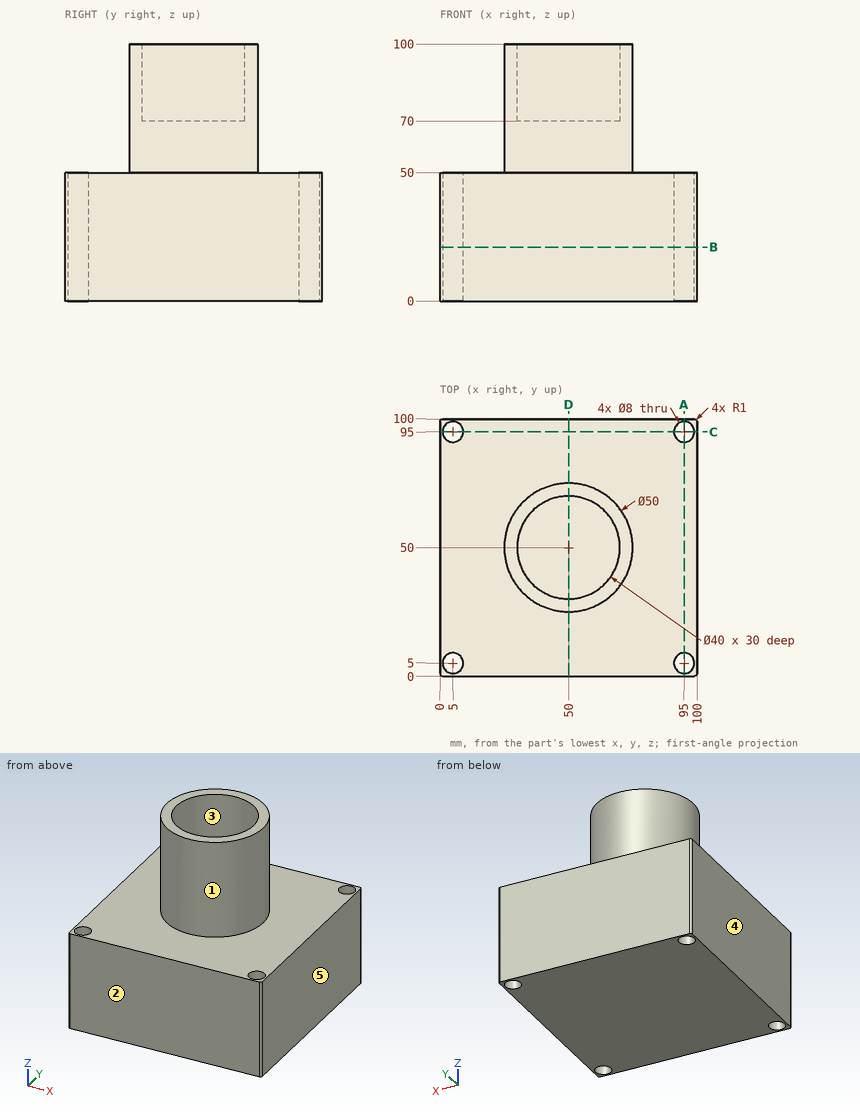
Geometry: see drawing. Coordinates: mm, zero at the bounding-box minimum. A direction names the side the tool comes from. Round coordinates to 2 decimals unless told otherwise and drop trailing zeros. Write each loop counter-clockwise with the first axis right and the second up, starting at its lowest first coordinate (ties: lowest second). Pieces come first, ordered by that corner, then holes.
1) Cut plane D-D (x = 50). Return the cut outline in (y, z), then the cut area to 3 significant figures.
2) Cut plane A-A (x = 95). Return the cut outline in (y, z).
3) Draft query along X for the marked faces 3, 4 and 5. Return one class per face: pulls with the +X half, pulls with the -X half, needs draft (parallel to the pull), parting line crosses it, or undercut.
4) Contact query for flat-ended pins moving along their axis: P1, Ø3, axis at x = 59.5, z = 67, coming from the +Y side; P2, Ø5, axis at x = 5, y = 95, coming from the -Z side; P3, Ø12, axis at y = 35, z = 89, coming from the +X side; P4, Ø3, axis at x = 39.5, y = 85.5, coming from the +Z side. Output: stop coordinate, or through.
5) Reachability of the marked faces 1 and 2 from +Z, -Z, +X, -X, +Y, -Y: full face, straight path, thin tool, end or side. Return the list, or none.
6) Cut plane B-B (z = 21). Return the cut outline in (x, y).
7) Ray query, L1, parallel to Y at x = 5, z = 17; L2, parallel to Y at x = 50, z = 89.75; L3, parallel to Z at x = 89, y = 69. Return the intervals inside material, ascending.
Geometry says:
1. outline: (0, 0) - (100, 0) - (100, 50) - (75, 50) - (75, 100) - (70, 100) - (70, 70) - (30, 70) - (30, 100) - (25, 100) - (25, 50) - (0, 50) - close
1. area: 6,300 mm2
2. outline: (0, 0) - (1, 0) - (1, 50) - (0, 50) - close; (9, 0) - (91, 0) - (91, 50) - (9, 50) - close; (99, 0) - (100, 0) - (100, 50) - (99, 50) - close
3. face 3: undercut
3. face 4: pulls with the -X half
3. face 5: pulls with the +X half
4. P1: stops at y = 73.69
4. P2: passes through
4. P3: stops at x = 73.32
4. P4: stops at z = 50
5. face 1: +Z
5. face 2: +Z, -Z, +X, -X, -Y
6. outline: (0, 1) arc R1 ccw to (1, 0) - (99, 0) arc R1 ccw to (100, 1) - (100, 99) arc R1 ccw to (99, 100) - (1, 100) arc R1 ccw to (0, 99) - close; hole circle Ø8 at (5, 5); hole circle Ø8 at (5, 95); hole circle Ø8 at (95, 5); hole circle Ø8 at (95, 95)
7. L1: y = 0 to 1, 9 to 91, 99 to 100
7. L2: y = 25 to 30, 70 to 75
7. L3: z = 0 to 50
